from build123d import *

# Parameters (mm, degrees)
F1_DEPTH = 9
F3_DEPTH = 10
F4_R     = 5


with BuildPart() as f1:
    # F0 (on Top) → F1 (new body, symmetric)
    with BuildSketch(Plane.XY):
        with BuildLine():
            ThreePointArc((42, -21.2), (43.2, -22.4), (44.4, -21.2))
            Line((44.4, -21.2), (44.4, -2.9))
            ThreePointArc((44.4, -2.9), (43.5506096654, -0.8493903346), (41.5, 0))
            Line((41.5, 0), (2.9, 0))
            ThreePointArc((2.9, 0), (0.8493903346, -0.8493903346), (0, -2.9))
            Line((0, -2.9), (0, -157.3))
            ThreePointArc((0, -157.3), (-0.0878679656, -157.5121320344), (-0.3, -157.6))
            Line((-0.3, -157.6), (-2.5, -157.6))
            ThreePointArc((-2.5, -157.6), (-2.7121320344, -157.5121320344), (-2.8, -157.3))
            Line((-2.8, -157.3), (-2.8, -151.6))
            ThreePointArc((-2.8, -151.6), (-2.5071067812, -150.8928932188), (-1.8, -150.6))
            Line((-1.8, -150.6), (-1.8, -148.2))
            Line((-1.8, -148.2), (-2.2, -148.2))
            ThreePointArc((-2.2, -148.2), (-4.3213203436, -149.0786796564), (-5.2, -151.2))
            Line((-5.2, -151.2), (-5.2, -157.3))
            ThreePointArc((-5.2, -157.3), (-4.4091883092, -159.2091883092), (-2.5, -160))
            Line((-2.5, -160), (-0.3, -160))
            ThreePointArc((-0.3, -160), (1.6091883092, -159.2091883092), (2.4, -157.3))
            Line((2.4, -157.3), (2.4, -2.9))
            ThreePointArc((2.4, -2.9), (2.5464466094, -2.5464466094), (2.9, -2.4))
            Line((2.9, -2.4), (41.5, -2.4))
            ThreePointArc((41.5, -2.4), (41.8535533906, -2.5464466094), (42, -2.9))
            Line((42, -2.9), (42, -21.2))
        make_face()
    extrude(amount=F1_DEPTH, both=True)

    # F2 (on Right) → F3 (cut, symmetric)
    with BuildSketch(Plane.YZ):
        with BuildLine():
            Line((-163, 4.75), (-145, 4.75))
            ThreePointArc((-145, 4.75), (-140.0502525317, 6.8002525317), (-138, 11.75))
            Line((-138, 11.75), (-168, 11.75))
            Line((-168, 11.75), (-168, -11.75))
            Line((-168, -11.75), (-138, -11.75))
            ThreePointArc((-138, -11.75), (-140.0502525317, -6.8002525317), (-145, -4.75))
            Line((-145, -4.75), (-163, -4.75))
            Line((-163, -4.75), (-163, 4.75))
        make_face()
    extrude(amount=F3_DEPTH, both=True, mode=Mode.SUBTRACT)

    # F4
    f4_edges = [f1.edges().sort_by_distance(p)[0] for p in [
        (1.2, -138.562803, 9),
        (1.2, -138.562803, -9),
    ]]
    fillet(f4_edges, radius=F4_R)


solid = f1.part
Source: CAD feature listing. Evaluate the final solid. Frame: model axes, mm. A direction names the side the tool comes from. Give positions to 0.01 mm unless a question says otherwise; leave off trailing zeros. Write each loop counter-clockwise with the first axis right and the second up, starting at its lowest first coordinate (ties: lowest second). Pieces come first, ordered by that corner, then holes. Notation, with made-up numbers: M -0.5,58 L 51.5,58 A18 ccw 51.5,93 Z; hole C 56,-35 d8. An arc over 180 degrees is marked long. Return JSON: item names as keys, results as strings. Group by question number.
1) Pull-direction query (Y, two-part tool) for faces 1 (the face through (-2.8, -154, 0)), 2 (the face through (0.3, -154.3, 4.75)), 3 (the face through (-4.3, -149.06, 0.07)); classes: pulls with the +Y half, pulls with the -Y half, needs draft (parallel to the pull), parting line crosses it, or undercut.
2) Set-up query: faces 4 (the face through (42, -12, 0)), 5 (the face through (0.3, -154.1, -4.75)), 6 (the face through (22, 0, 0)). Return all of +Z, -Z, +X, -X, +Y, -Y with unobstructed straight access to the full face (end or side cutting, diameter ignored); none if empty.
3) Pin query (flat end, axial travel): P1, Ø0.7, axis at y = -149, z = 1.5, coming from the +X side; P2, Ø6, axis at x = -1.5, y = -150, coming from the -Z side; P3, Ø6, axis at x = -2, y = -153, coming from the +Z side. Return the tip coordinate at first contact, or that it passes through.
4) Cut plane B-B, the plane y = -115.5. Output: boundary loops of the cut face in (x, z), plus the area to 3 significant figures.
5) Cut plane A-A, the plane z = -3. Output: boundary loops of the cut face in (x, y), plus the area to 3 significant figures.
6) Material intervals for line 1 along X through (y, z) = (-12.5, 4); line 2 along Y through (x, z) = (32, 2); line 3 along X through (y, z) = (-41.5, -8), sorted ascending. Write a range as [from, to].
7) Cut plane C-C, the plane x = 20. Output: boundary loops of the cut face in (y, z), plus the area to 3 significant figures.
Recorded:
{
 "1": {"face 1": "undercut", "face 2": "needs draft", "face 3": "pulls with the +Y half"},
 "2": {"face 4": "+Z, -Z, -Y", "face 5": "-Z, +X, -X, -Y", "face 6": "+Z, -Z, +X, -X, +Y"},
 "3": {"P1": "stops at x = 2.4", "P2": "stops at z = -4.75", "P3": "stops at z = 4.75"},
 "4": {"outline": "M 0,-9 L 2.4,-9 L 2.4,9 L 0,9 Z", "area": "43.2 mm²"},
 "5": {"outline": "M -5.2,-157.3 A2.7 ccw -2.5,-160 L -0.3,-160 A2.7 ccw 2.4,-157.3 L 2.4,-2.9 A0.5 cw 2.9,-2.4 L 41.5,-2.4 A0.5 cw 42,-2.9 L 42,-21.2 A1.2 ccw 44.4,-21.2 L 44.4,-2.9 A2.9 ccw 41.5,0 L 2.9,0 A2.9 ccw 0,-2.9 L 0,-157.3 A0.3 cw -0.3,-157.6 L -2.5,-157.6 A0.3 cw -2.8,-157.3 L -2.8,-151.6 A1 cw -1.8,-150.6 L -1.8,-148.2 L -2.2,-148.2 A3 ccw -5.2,-151.2 Z", "area": "561 mm²"},
 "6": {"line 1": "x = [0, 2.4], [42, 44.4]", "line 2": "y = [-2.4, 0]", "line 3": "x = [0, 2.4]"},
 "7": {"outline": "M -2.4,-9 L 0,-9 L 0,9 L -2.4,9 Z", "area": "43.2 mm²"}
}
